from build123d import *

# Parameters (mm, degrees)
SKETCH1_R           = 2.1
BOSS_EXTRUDE1_DEPTH = 4
SKETCH2_W           = 80
SKETCH2_H           = 5
BOSS_EXTRUDE2_DEPTH = 36
SKETCH3_W           = 5
SKETCH3_H           = 40
BOSS_EXTRUDE3_DEPTH = 61
SKETCH4_W           = 80
SKETCH4_H           = 66
BOSS_EXTRUDE4_DEPTH = 5
CHAMFER2_SIZE       = 1
SKETCH5_R           = 1.35
CUT_EXTRUDE1_DEPTH  = 5


with BuildPart() as part:
    # Sketch1 → Boss-Extrude1 (new body)
    with BuildSketch(Plane(origin=(0, 0, 0), x_dir=(1, 0, 0), z_dir=(0, 1, 0))):
        with BuildLine():
            Line((-58.8413396, 11.682242991), (52.1586604, 11.682242991))
            ThreePointArc((52.1586604, 11.682242991), (55.694194306, 10.217776897), (57.1586604, 6.682242991))
            Line((57.1586604, 6.682242991), (57.1586604, 0.682242991))
            ThreePointArc((57.1586604, 0.682242991), (55.694194306, -2.853290915), (52.1586604, -4.317757009))
            Line((52.1586604, -4.317757009), (-63.8413396, -4.317757009))
            Line((-63.8413396, -4.317757009), (-63.8413396, 6.682242991))
            ThreePointArc((-63.8413396, 6.682242991), (-62.376873506, 10.217776897), (-58.8413396, 11.682242991))
        make_face()
        with Locations((-58.8413396, 6.682242991)):
            Circle(SKETCH1_R, mode=Mode.SUBTRACT)
        with Locations((39.1586604, 1.682242991)):
            Circle(SKETCH1_R, mode=Mode.SUBTRACT)
        with Locations((49.1586604, 1.682242991)):
            Circle(SKETCH1_R, mode=Mode.SUBTRACT)
    extrude(amount=BOSS_EXTRUDE1_DEPTH)

    # Sketch2 → Boss-Extrude2 (add)
    with BuildSketch(Plane(origin=(0, 4, 0), x_dir=(1, 0, 0), z_dir=(0, 1, 0))):
        with Locations((-23.8413396, -1.817757009)):
            Rectangle(SKETCH2_W, SKETCH2_H)
    extrude(amount=BOSS_EXTRUDE2_DEPTH)

    # Sketch3 → Boss-Extrude3 (add)
    with BuildSketch(Plane.XY.offset(4.317757009)):
        with Locations((-61.3413396, 20)):
            Rectangle(SKETCH3_W, SKETCH3_H)
    extrude(amount=BOSS_EXTRUDE3_DEPTH)

    # Sketch4 → Boss-Extrude4 (add)
    with BuildSketch(Plane(origin=(0, 40, 0), x_dir=(1, 0, 0), z_dir=(0, 1, 0))):
        with Locations((-23.8413396, -32.317757009)):
            Rectangle(SKETCH4_W, SKETCH4_H)
    extrude(amount=BOSS_EXTRUDE4_DEPTH)

    # Chamfer2
    chamfer2_edges = [part.edges().sort_by_distance(p)[0] for p in [
        (55.694194306, 4, 2.853290915),
        (-60.9413396, 4, -6.682242991),
        (57.1586604, 4, -3.682242991),
        (37.0586604, 4, -1.682242991),
        (55.694194306, 4, -10.217776897),
        (47.0586604, 4, -1.682242991),
        (-3.3413396, 4, -11.682242991),
        (34.1586604, 4, 4.317757009),
        (-63.8413396, 24.5, -0.682242991),
        (16.1586604, 4, 1.817757009),
        (16.1586604, 22, 4.317757009),
        (-23.8413396, 4, -0.682242991),
        (16.1586604, 24.5, -0.682242991),
        (-62.376873506, 4, -10.217776897),
        (-63.8413396, 22.5, 65.317757009),
        (-58.8413396, 20, 65.317757009),
        (-21.3413396, 40, 65.317757009),
        (16.1586604, 40, 34.817757009),
        (16.1586604, 42.5, 65.317757009),
        (-63.8413396, 45, 32.317757009),
        (-23.8413396, 45, 65.317757009),
        (16.1586604, 45, 32.317757009),
        (-23.8413396, 45, -0.682242991),
        (-63.8413396, 4, -3.682242991),
    ]]
    chamfer(chamfer2_edges, length=CHAMFER2_SIZE)

    # Sketch5 → Cut-Extrude1 (cut)
    with BuildSketch(Plane(origin=(0, 45, 0), x_dir=(1, 0, 0), z_dir=(0, 1, 0))):
        with Locations((11.1586604, -4.317757009)):
            Circle(SKETCH5_R)
        with Locations((-58.8413396, -4.317757009)):
            Circle(SKETCH5_R)
        with Locations((-58.8413396, -14.317757009)):
            Circle(SKETCH5_R)
        with Locations((11.1586604, -14.317757009)):
            Circle(SKETCH5_R)
        with Locations((-58.8413396, -24.317757009)):
            Circle(SKETCH5_R)
        with Locations((11.1586604, -24.317757009)):
            Circle(SKETCH5_R)
        with Locations((-58.8413396, -34.317757009)):
            Circle(SKETCH5_R)
        with Locations((11.1586604, -34.317757009)):
            Circle(SKETCH5_R)
        with Locations((-58.8413396, -44.317757009)):
            Circle(SKETCH5_R)
        with Locations((11.1586604, -44.317757009)):
            Circle(SKETCH5_R)
        with Locations((-58.8413396, -54.317757009)):
            Circle(SKETCH5_R)
        with Locations((11.1586604, -54.317757009)):
            Circle(SKETCH5_R)
    extrude(amount=-CUT_EXTRUDE1_DEPTH, mode=Mode.SUBTRACT)


solid = part.part
Source: CAD feature listing. Evaluate the final solid. Frame: model axes, mm. A direction names the side the tool comes from. Give positions to 0.01 mm unless a question says otherwise; leave off trailing zeros. Write each loop counter-clockwise with the first axis right and the second up, starting at its lowest first coordinate (ties: lowest second). Pieces come first, ordered by that corner, then holes. Notation, with made-up numbers: M 47,32 L 80,32 A19 cw 80,64 Z; hole C -28,39.25 d9. An arc over 180 degrees is marked long. Answer as a JSON object with one key per item and string values.
Q1. Cut plane B-B, the plane y = 38. Return the cut outline in (x, z), then the cut area to 4 significant figures.
Geometry check:
{"outline": "M -63.84,0.32 L -62.84,-0.68 L 15.16,-0.68 L 16.16,0.32 L 16.16,3.32 L 15.16,4.32 L -58.84,4.32 L -58.84,64.32 L -59.84,65.32 L -62.84,65.32 L -63.84,64.32 Z", "area": "702.5 mm^2"}
Q2. Cut plane C-C, the plane z = 21. Return the cut outline in (x, y), then the cut area to 4 significant figures.
Geometry check:
{"outline": "M -63.84,0 L -58.84,0 L -58.84,40 L 15.16,40 L 16.16,41 L 16.16,44 L 15.16,45 L -62.84,45 L -63.84,44 Z", "area": "598.5 mm^2"}
Q3. Contact query for flat-ended pins moving along their axis: P1, Ø2, axis at x = -58.84, z = 4.32, coming from the +Y side; P2, Ø8, axis at y = 37.5, z = 0, coming from the +X side; P3, Ø11.5, axis at y = 16.5, z = 38.5, coming from the +X side. Output: stop coordinate, or through.
Geometry check:
{"P1": "stops at y = 40", "P2": "stops at x = 16.16", "P3": "stops at x = -58.84"}
Q4. Access query for faces 1 (the face through (-58.841, 20, 34)), 2 (the face through (-57.554, 42.535, 53.912)), 3 (the face through (-63.841, 22, 29)). Directions: +Z, -Z, +X, -X, +Y, -Y. A direction counts if a zero-diameter tool reaches every point of the face in a straight line with its end or side. Return the directions, or none.
Geometry check:
{"face 1": "+Z, +X, -Y", "face 2": "+Y", "face 3": "+Z, -Z, -X, +Y, -Y"}
Q5. Ray query, line 1 along Z through (x, y) = (-8, 5.5); line 2 along X through (y, z) = (16, 30); line 3 along X through (y, z) = (40.5, 21). Return the intervals inside material, ascending.
Geometry check:
{"line 1": "z = -0.68 to 4.32", "line 2": "x = -63.84 to -58.84", "line 3": "x = -63.84 to 15.66"}
Q6. Cut plane A-A, the plane x = -23. Return the cut outline in (y, z).
Geometry check:
{"outline": "M 0,-11.68 L 3,-11.68 L 4,-10.68 L 4,-1.68 L 5,-0.68 L 44,-0.68 L 45,0.32 L 45,64.32 L 44,65.32 L 41,65.32 L 40,64.32 L 40,4.32 L 0,4.32 Z"}
Q7. Mould query, pull axis Z, two halves, no side actions, for faces 4 (the face through (-57.594, 42.535, 14.835)), 5 (the face through (-4, 1, -11.682)), 6 (the face through (-3, 4, -5)). Classes: +Z half, -Z half, draft (parallel to the pull), parting line (faces both ways), or undercut.
Geometry check:
{"face 4": "undercut", "face 5": "-Z half", "face 6": "draft"}
